Geometry check sheet. Reference: drawing and pictorial views, mm from the part's lowest x, y, z. A direction names the side the tool comes from. Give positions to 0.01 mm unless a question says otherwise; leave off trailing zeros. Loops run counter-clockwise (first coordinate to the right, second up) from the corner with the lowest first, then second, coordinate; pieces in that order, holes last. Notation, with made-up numbers: M 16.5,87 L 53.5,87 A23 ccw 53.5,97 Z; hole C 51,83.5 d4. An arc over 180 degrees is marked long. Put each result on its own line as item: value. Start each with the question number.
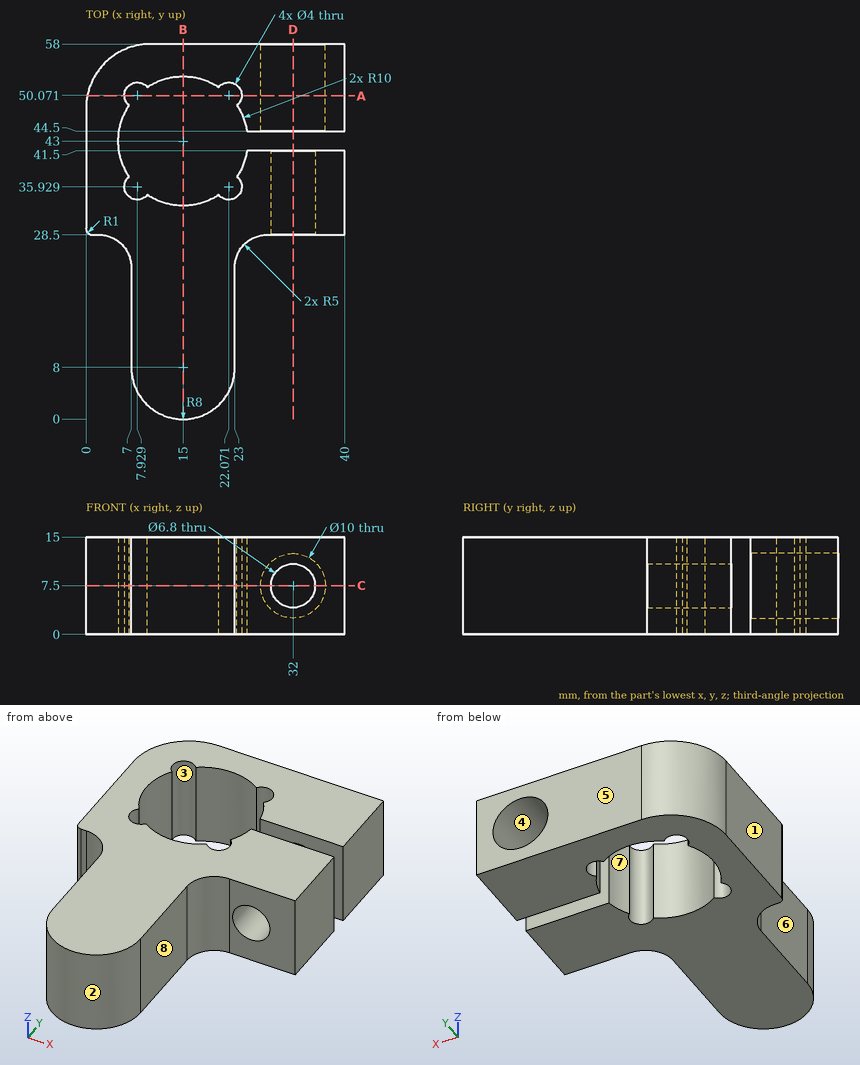
Q1. Section check D-D, the plane x = 32. Record the cut outline in (y, z), then the cut area to 3 significant figures.
Q2. Section check A-A, the plane y = 50. Record the cut outline in (x, z), then the cut area to 3 significant figures.
Q3. Section check B-B, the plane x = 15. Record the cut outline in (y, z).
Q4. Section check C-C, the plane z = 7.5. Give the number of separate pieces and of enclosed holes in the cut face, then the cut area to 3 significant figures.
Q5. Mould release check, pull along Y, two halves, no side actions. Record for the marked faces 1, 2 and 3: pulls with the +Y half, pulls with the -Y half, needs draft (parallel to the pull), parting line crosses it, or undercut.
Q6. Depth check by flat-ended pin: P1, Ø0.5, axis at x = 1.5, z = 5, coming from the -Y side; P2, Ø4.5, axis at y = 18.5, z = 11, coming from the -X side; P3, Ø4.5, axis at y = 15, z = 4.5, coming from the +X side. Enter the tip coordinate at first touch or a pass-through.
Q7. Thickness scan on line 1 along Y through (x, z) = (35, 11.75); line 2 along Z through (x, y) = (32, 32); line 3 along Y through (x, z) = (32.5, 3.75). Record the ranges inside material, lowest first. Write a range as [from, to].
Q8. Access from +Z, -Z, +X, -X, +Y, -Y to the whole of each face (thin tool, end or side, straight path). Record for the marked faces 4, 5, 6, 7 and 8.
Found:
1. outline: M 28.5,0 L 41.5,0 L 41.5,4.1 L 28.5,4.1 Z; M 28.5,10.9 L 41.5,10.9 L 41.5,15 L 28.5,15 Z; M 44.5,0 L 58,0 L 58,2.5 L 44.5,2.5 Z; M 44.5,12.5 L 58,12.5 L 58,15 L 44.5,15 Z
1. area: 174 mm^2
2. outline: M 0.2,0 L 5.93,0 L 5.93,15 L 0.2,15 Z; M 24.07,0 L 40,0 L 40,15 L 24.07,15 Z; hole C 32,7.5 d10
2. area: 246 mm^2
3. outline: M 0,0 L 33,0 L 33,15 L 0,15 Z; M 53,0 L 58,0 L 58,15 L 53,15 Z
4. separate pieces: 3
4. enclosed holes: 0
4. area: 989 mm^2
5. face 1: needs draft
5. face 2: pulls with the -Y half
5. face 3: undercut
6. P1: stops at y = 28.5
6. P2: stops at x = 7
6. P3: stops at x = 23
7. line 1: y = [28.5, 41.5], [44.5, 58]
7. line 2: z = [0, 4.1], [10.9, 15]
7. line 3: y = [28.5, 41.5]
8. face 4: +Y
8. face 5: +Z, -Z, +X, -X, +Y
8. face 6: +Z, -Z, -X, -Y
8. face 7: +Z, -Z
8. face 8: +Z, -Z, +X, -Y
